Job drawing, mm, ordinate dimensions from the low corner. One solid piece. A direction names the side the tool comes from. Give positions to 0.01 mm unless a question says otherwise; leave off trailing zeros. Write each loop counter-clockwise with the first axis right and the second up, starting at its lowest first coordinate (ties: lowest second). Pieces come first, ordered by that corner, then holes. Notation, with made-up numbers: M -30,-19 L 22,-19 A26 cw 22,10 Z; hole C -25.5,40.5 d10. An arc over 180 degrees is marked long. Use CSV: the item, a comma, the result in double quotes. Start each with the question number.
Item 1: Cut at C-C (y = 6). List the corners of the cut face in (x, z), then the cut area to 3 significant figures.
Item 2: Cut at A-A (z = 35). List the corners of the cut face in (x, y).
Item 3: Drill centre lines: line 1 (Z direction, x = 35, y = 1.2); line 2 (X direction, y = 3.5, z = 36); line 3 (Y direction, x = 16.5, z = 42.5). Where is each one in solid material? Low to high. Write a range as [from, to].
Item 4: Cut at D-D (z = 65). List the corners of the cut face in (x, y), then the cut area to 3 significant figures.
Item 5: Mould opens along Z. For the marked faces 3 and 4 say: released by +Z, released by -Z, zero draft, split by the parting line, or undercut.
Item 6: Pin check, flat tips, straight feed: pin 1 (9 mm diameter, centred on x = 65, z = 35, fed in from -Y); pin 2 (7 mm diameter, centred on x = 5, z = 35, fed in from +Y); pin 3 (1.5 mm diameter, centred on x = 36, z = 44, fed in from -Y); pin 4 (1.5 mm diameter, centred on y = 3.5, z = 39.5, fed in from +X). Stop position of each tip, or through.
Item 7: Cut at B-B (x = 5). List the corners of the cut face in (y, z).
Item 8: Which spindle directions (+Z, -Z, +X, -X, +Y, -Y) get a long thin tool onto all of the face, cutting with end or side? Do the marked faces 1 and 2. Say none if no direction does.
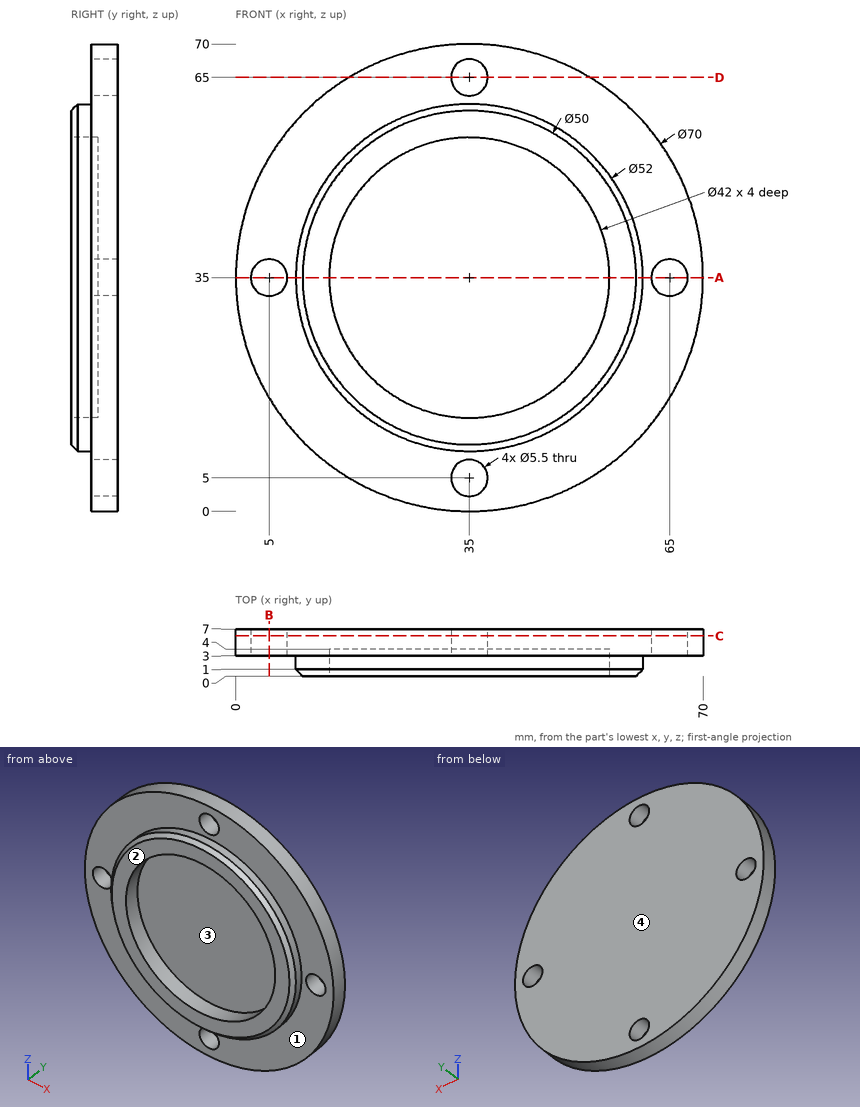
Worked answers:
1,outline,"C 35,35 d70; hole C 5,35 d5.5; hole C 35,5 d5.5; hole C 35,65 d5.5; hole C 65,35 d5.5"
1,area,"3,750 mm^2"
2,outline,"M 0,3 L 2.25,3 L 2.25,7 L 0,7 Z; M 7.75,3 L 9,3 L 9,1 L 10,0 L 14,0 L 14,4 L 56,4 L 56,0 L 60,0 L 61,1 L 61,3 L 62.25,3 L 62.25,7 L 7.75,7 Z; M 67.75,3 L 70,3 L 70,7 L 67.75,7 Z"
3,line 1,"z = [9, 14], [56, 61]"
3,line 2,"x = [0.01, 2.44], [7.56, 14.02], [55.98, 62.44], [67.56, 69.99]"
3,line 3,"y = [4, 7]"
4,outline,"M 16.97,3 L 32.25,3 L 32.25,7 L 16.97,7 Z; M 37.75,3 L 53.03,3 L 53.03,7 L 37.75,7 Z"
4,area,"122 mm^2"
5,face 3,"undercut"
5,face 4,"zero draft"
6,pin 1,"stops at y = 0.5"
6,pin 2,"stops at y = 7"
6,pin 3,"stops at y = 4"
6,pin 4,"stops at x = 69.8"
7,outline,"M 3,16.97 L 7,16.97 L 7,32.25 L 3,32.25 Z; M 3,37.75 L 7,37.75 L 7,53.03 L 3,53.03 Z"
8,face 1,"-Y"
8,face 2,"+Z, -Z, +X, -X, -Y"
